Answer from the drawing. Dimensions are ordinates in mm from the lowest x, y and z of the part. A direction names the side the tool comes from. Give positions to 0.01 mm unless a question says otherwise; leave off trailing zeros. Write each question's results on one line, items separated by ' | '. Start each with the question number.
Item 1: Which of the six approach directions +Z, -Z, +X, -X, +Y, -Y give full straight-line access (tool end or side, diameter ignored) to the marked faces 4 and 5?
Item 2: Determine the mould class of the marked faces 1, 2 and 3 for opening direction Y: +Y half, -Y half, draft (parallel to the pull), parting line (faces both ways), or undercut.
Item 3: Each of these flat-tipped pins is pushed along its axis until it touches: P1, Ø8, axis at y = 5.5, z = 21, coming from the +X side; P2, Ø2, axis at y = 1.5, z = 7, coming from the +X side; P3, Ø1.3, axis at x = 4, z = 6, coming from the -Y side; P4, Ø2, axis at x = 1.5, z = 12.5, coming from the -Y side. Where does it stop, or does it pass through?
Item 4: Find the intervals of material crossed by line 1 (Y direction, x = 3, z = 1.5) (1 decimal); line 2 (Y direction, x = 4, z = 4.75) (1 decimal); line 3 (Z direction, x = 6, y = 44), in increasing order.
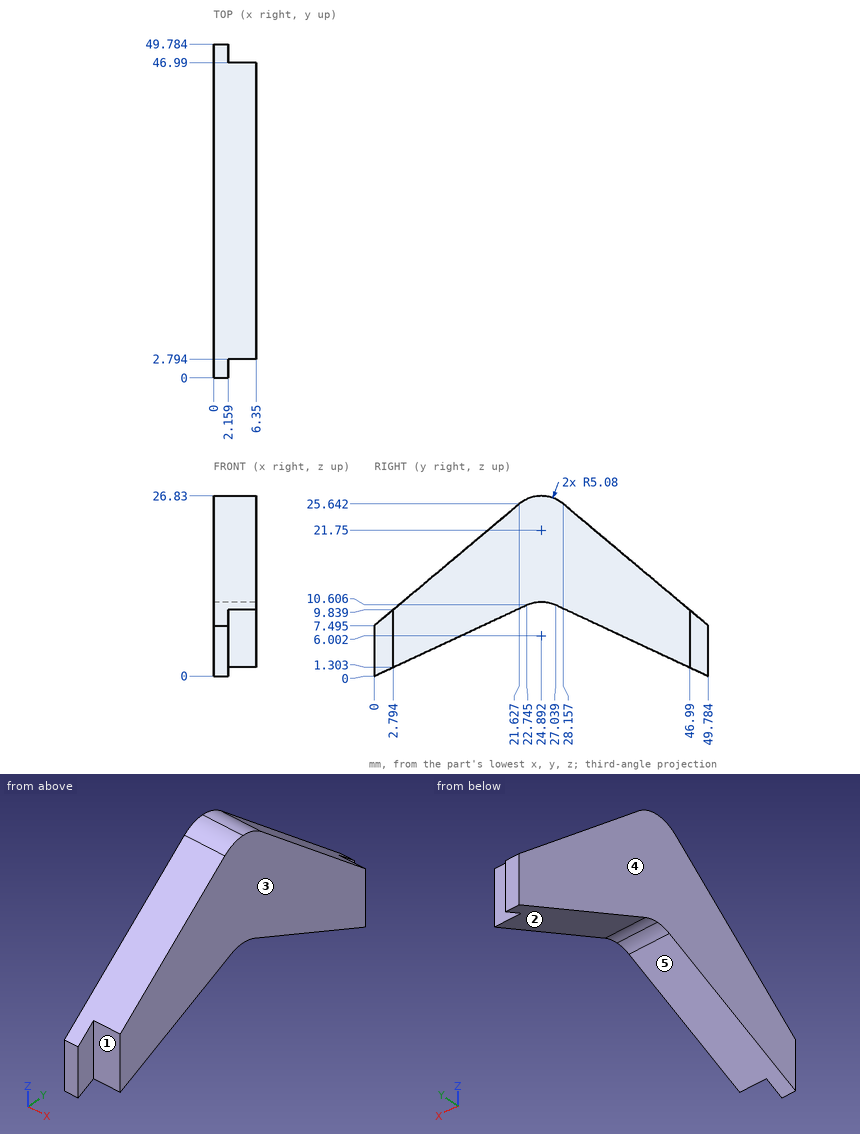
Findings:
1) face 4: +Z, -Z, -X, +Y, -Y | face 5: -Z, +X, -X
2) face 1: -Y half | face 2: undercut | face 3: draft
3) P1: through | P2: x = 2.16 | P3: y = 2.79 | P4: y = 4.77
4) line 1: 2.8 to 3.2, 46.6 to 47 | line 2: 2.8 to 10.2, 39.6 to 47 | line 3: 2.7 to 12.35
